Geometry: final body of the model. Coordinates: model frame, mm. A direction names the side the tool comes from. Give positions to 0.01 mm unless a question says otherwise; leave off trailing zeros. Order: outer loops, then holes, each group sorted by start corner. A loop starts at its lowest first (then second) coordinate and runs counter-clockwise, first axis right, second up. Notation, with made-up numbers: (-35, -7.5) -> (-13, -7.5) arc R32 cw to (-13, 28.5) -> close; hole circle Ø3 at (-11.75, 54). An arc over 180 degrees is marked (long way). Answer in a Markdown table with one row per item. Add a question column.
Q1. Line query: line 1 along Y through (x, z) = (92, 2.7); line 2 along Y through (x, z) = (249.5, 2.75); line 3 along Y through (x, z) = (25, 4.45) (3 decimals). Output: solid intervals per line, ascending. Write a range as from..to.
Q2. Pull-direction query (X, two-part tool) for faces 5 (the face through (0, 12, 2)), 6 (the face through (247, 0, 2)), 7 (the face through (152.609, 47.846, 2.317)); classes: +X half, -X half, draft (parallel to the pull), parting line (faces both ways), or undercut.
Q3. Set-up query: faces 1 (the face through (111, 4.699, 2)), 2 (the face through (23, 4.699, 2)), 3 (the face through (271, 67.733, 2)), 4 (the face through (150, 19.172, 2)). Return all of +Z, -Z, +X, -X, +Y, -Y with unobstructed straight access to the full face (end or side cutting, diameter ignored); none if empty.
Q4. Cut plane C-C on x = 204. Return the cut outline in (y, z), and give its area (3 significant figures).
Q5. Cut plane B-B on y = 29. Return the cut outline in (x, z), and give its area (3 significant figures).
Q6. Cut plane D-D on y = 83. Return the cut outline in (x, z).
Q7. Contact query for flat-ended pins moving along their axis: P1, Ø2.5, axis at y = 56.5, z = 2, coming from the +X side; P2, Ø2.5, axis at x = 14, z = 1.5, coming from the -Y side; P3, Ø1.4, axis at y = 2.5, z = 2, coming from the -X side; P4, Ø5, axis at x = 146.5, y = 23.5, coming from the +Z side. Output: stop coordinate, or through.
Q8. Cut plane A-A on z = 1.6. Return the cut outline in (x, y).
from build123d import *

# Parameters (mm, degrees)
BOSS_EXTRUDE1_DEPTH = 4.699
SKETCH2_W           = 44.45
SKETCH2_H           = 4.699
CUT_EXTRUDE1_DEPTH  = 288.196060581
CAVITY3_START       = 268.350970906
CAVITY3_OUTLINE_W   = 21.166666666
CAVITY3_OUTLINE_H   = 4.699
CAVITY3_DEPTH       = 4.699


# Read off the part's stored shape, not the designer's step: Cavity3
with BuildPart() as part:
    # Sketch1 → Boss-Extrude1 (new body)
    with BuildSketch(Plane.XY):
        Polygon((273.049970906, 58.684987569), (273.049970906, 88.9), (253.999970906, 88.9), (0, 19.05), (0, 0), (273.049970906, 0), (273.049970906, 30.215012431), align=None)
        Polygon((48.33831711, 19.171571116), (253.999970906, 19.171571116), (253.999970906, 75.728532388), align=None, mode=Mode.SUBTRACT)
    extrude(amount=BOSS_EXTRUDE1_DEPTH)

    # Sketch2 → Cut-Extrude1 (cut, through all)
    with BuildSketch(Plane(origin=(0, 0, 0), x_dir=(-1, 0, 0), z_dir=(0, 0, -1))):
        with Locations((-22.225, 2.3495)):
            Rectangle(SKETCH2_W, SKETCH2_H)
        with Locations((-111.125, 2.3495)):
            Rectangle(SKETCH2_W, SKETCH2_H)
        with Locations((-200.025, 2.3495)):
            Rectangle(SKETCH2_W, SKETCH2_H)
    extrude(amount=-CUT_EXTRUDE1_DEPTH, mode=Mode.SUBTRACT)

    # Cavity3 outline → Cavity3 (cut)
    with BuildSketch(Plane.YZ.offset(CAVITY3_START)):
        with Locations((57.15, 2.3495)):
            Rectangle(CAVITY3_OUTLINE_W, CAVITY3_OUTLINE_H)
    extrude(amount=CAVITY3_DEPTH, mode=Mode.SUBTRACT)


solid = part.part
Completed:
| question | item | result |
|---|---|---|
| 1 | line 1 | y = 4.7..19.17, 31.18..44.35 |
| 1 | line 2 | y = 0..19.17, 74.49..87.66 |
| 1 | line 3 | y = 4.699..25.925 |
| 2 | face 5 | -X half |
| 2 | face 6 | draft |
| 2 | face 7 | undercut |
| 3 | face 1 | +Z, -Z, -Y |
| 3 | face 2 | +Z, -Z, -X, -Y |
| 3 | face 3 | +Z, -Z, +X |
| 3 | face 4 | +Z, -Z |
| 4 | outline | (4.7, 0) -> (19.17, 0) -> (19.17, 4.7) -> (4.7, 4.7) -> close; (61.98, 0) -> (75.15, 0) -> (75.15, 4.7) -> (61.98, 4.7) -> close |
| 4 | area | 130 mm² |
| 5 | outline | (36.18, 0) -> (84.08, 0) -> (84.08, 4.7) -> (36.18, 4.7) -> close; (254, 0) -> (273.05, 0) -> (273.05, 4.7) -> (254, 4.7) -> close |
| 5 | area | 315 mm² |
| 6 | outline | (232.55, 0) -> (273.05, 0) -> (273.05, 4.7) -> (232.55, 4.7) -> close |
| 7 | P1 | stops at x = 268.35 |
| 7 | P2 | stops at y = 4.7 |
| 7 | P3 | stops at x = 44.45 |
| 7 | P4 | passes through |
| 8 | outline | (0, 4.7) -> (44.45, 4.7) -> (44.45, 0) -> (88.9, 0) -> (88.9, 4.7) -> (133.35, 4.7) -> (133.35, 0) -> (177.8, 0) -> (177.8, 4.7) -> (222.25, 4.7) -> (222.25, 0) -> (273.05, 0) -> (273.05, 46.57) -> (268.35, 46.57) -> (268.35, 67.73) -> (273.05, 67.73) -> (273.05, 88.9) -> (254, 88.9) -> (0, 19.05) -> close; hole (48.34, 19.17) -> (254, 19.17) -> (254, 75.73) -> close |
